```python
from build123d import *

# Parameters (mm, degrees)
ESQUISSE1_W                  = 52
ESQUISSE1_H                  = 3
CHANFREIN1_SIZE              = 0.5
ENL_V_MAT_EXTRU_1_DEPTH      = 27.343879745
ENL_V_MAT_EXTRU_1_DEPTH_BACK = 27.343879745
ESQUISSE2_W                  = 4
ESQUISSE2_H                  = 2
ESQUISSE3_W                  = 0.74
ESQUISSE3_H                  = 1
BOSS_EXTRU_1_START           = 15
ESQUISSE4_R                  = 3
BOSS_EXTRU_1_DEPTH           = 15
ENL_V_MAT_EXTRU_2_DEPTH      = 42.218927691
ENL_V_MAT_EXTRU_2_DEPTH_BACK = 42.218927691
ESQUISSE5_W                  = 12
ESQUISSE5_H                  = 1
ENL_V_MAT_EXTRU_3_DEPTH      = 42.218927691
ENL_V_MAT_EXTRU_3_DEPTH_BACK = 42.218927691
ESQUISSE6_W                  = 50.211323454
ESQUISSE6_H                  = 20.21753951


with BuildPart() as part:
    # Esquisse1 → Révolution1 (revolve)
    with BuildSketch(Plane.XY, mode=Mode.PRIVATE) as r_volution1_sk:
        with Locations((0, 1.5)):
            Rectangle(ESQUISSE1_W, ESQUISSE1_H)
    revolve(r_volution1_sk.sketch.rotate(Axis((0, 0, 0), (1, 0, 0)), 90), axis=Axis((0, 0, 0), (1, 0, 0)))

    # Chanfrein1
    chanfrein1_edges = [part.edges().sort_by_distance(p)[0] for p in [
        (26, 0, -3),
    ]]
    chamfer(chanfrein1_edges, length=CHANFREIN1_SIZE)

    # Esquisse2 → Enlèv. mat.-Extru.1 (cut, two sides: drawn at the far end of the back side and taken through both)
    with BuildSketch(Plane.XY.offset(-ENL_V_MAT_EXTRU_1_DEPTH_BACK)):
        with Locations((9.5, 3)):
            Rectangle(ESQUISSE2_W, ESQUISSE2_H)
    extrude(amount=ENL_V_MAT_EXTRU_1_DEPTH + ENL_V_MAT_EXTRU_1_DEPTH_BACK, mode=Mode.SUBTRACT)

    # Esquisse3 → Enlèvement de matière-Révolution1 (revolve, cut)
    with BuildSketch(Plane.XY):
        with Locations((-21.03, 2.5)):
            Rectangle(ESQUISSE3_W, ESQUISSE3_H)
        with Locations((21.03, 2.5)):
            Rectangle(ESQUISSE3_W, ESQUISSE3_H)
    revolve(axis=Axis((0, 0, 0), (-1, 0, 0)), mode=Mode.SUBTRACT)

    # Esquisse4 → Boss.-Extru.1 (add)
    with BuildSketch(Plane.ZY.offset(26).offset(BOSS_EXTRU_1_START)):
        with Locations(Location((0, 0, 0), (0, 0, 90))):
            Circle(ESQUISSE4_R)
    extrude(amount=-BOSS_EXTRU_1_DEPTH)

    # Esquisse5 → Enlèv. mat.-Extru.2 (cut, two sides: drawn at the far end of the back side and taken through both)
    with BuildSketch(Plane.XY.offset(-ENL_V_MAT_EXTRU_2_DEPTH_BACK)):
        with Locations((-35, 2.5)):
            Rectangle(ESQUISSE5_W, ESQUISSE5_H)
    extrude(amount=ENL_V_MAT_EXTRU_2_DEPTH + ENL_V_MAT_EXTRU_2_DEPTH_BACK, mode=Mode.SUBTRACT)

    # Esquisse6 → Enlèv. mat.-Extru.3 (cut, two sides: drawn at the far end of the back side and taken through both)
    with BuildSketch(Plane.XY.offset(-ENL_V_MAT_EXTRU_3_DEPTH_BACK)):
        with Locations((-25.105661727, 1.097333559)):
            Rectangle(ESQUISSE6_W, ESQUISSE6_H)
    extrude(amount=ENL_V_MAT_EXTRU_3_DEPTH + ENL_V_MAT_EXTRU_3_DEPTH_BACK, mode=Mode.SUBTRACT)


solid = part.part
```
The listing builds one solid part. Answer for the finished solid, in the listing's coordinates (mm). A direction names the side the tool comes from. Coordinates: 2 decimals unless noted, no trailing zeros. Write each loop counter-clockwise with the first axis right and the second up, starting at its lowest first coordinate (ties: lowest second). Pieces come first, ordered by that corner, then holes.
Q1. Section B-B, the plane x = 17 is taken. Write down the section's boundary in (y, z).
Returned:
outline: circle Ø6 at (0, 0)
Q2. Given P1, Ø1.5, axis at x = 12, y = 1, coming from the -Z side; P2, Ø3, axis at y = 1, z = 0.5, coming from the -X side; P3, Ø2, axis at x = 10, z = 1, coming from the +Y side; P4, Ø2, axis at x = 22.5, y = -2, coming from the -Z side, each flat-ended and moving along its own axis, determine where each tip first touches the part or whether it passes through.
Returned:
P1: stops at z = -2.99
P2: stops at x = 0
P3: stops at y = 2
P4: stops at z = -2.83
Q3. Section C-C, the plane x = 10 is taken. Write down the section's boundary in (y, z), then the cut area to 3 significant figures.
Returned:
outline: (2, -2.24) - (2, 2.24) arc R3 ccw (long way) to start
area: 25.2 mm2
Q4. Section A-A, the plane z = 0 is taken. Write down the section's boundary in (x, y).
Returned:
outline: (0, -3) - (20.66, -3) - (20.66, -2) - (21.4, -2) - (21.4, -3) - (25.5, -3) - (26, -2.5) - (26, 2.5) - (25.5, 3) - (21.4, 3) - (21.4, 2) - (20.66, 2) - (20.66, 3) - (11.5, 3) - (11.5, 2) - (7.5, 2) - (7.5, 3) - (0, 3) - close
Q5. Which of the six approach directions +Z, -Z, +X, -X, +Y, -Y give full straight-line access (tool end or side, diameter ignored) to faces 5 (the flat face through (11.5, 2.4, 0)), 6 (the cylindrical face through (23.48, 1.15, 2.77)), 7 (the cylindrical face through (21, 0, 2))?
Returned:
face 5: +Z, -Z, +Y
face 6: +X, -X
face 7: none
Q6. The mould has two halves that part along X. Classify faces 1 (the flat face through (20.66, -1, 2)), 2 (the flat face through (0, 0, 0)), 3 (the flat face through (26, 0, 0)), 4 (the cylindrical face through (10, -3, 0)): released by +X, released by -X, zero draft, split by the parting line, or undercut.
Returned:
face 1: undercut
face 2: released by -X
face 3: released by +X
face 4: zero draft
Q7. Find the intervals of material crossed by line 1 along X through (y, z) = (-0.2, -2.3); line 2 along X through (y, z) = (-0.1, -2.6); line 3 along Z through (x, y) = (5.25, 1.5), in increasing order.
Returned:
line 1: x = 0 to 20.66, 21.4 to 26
line 2: x = 0 to 20.66, 21.4 to 25.9
line 3: z = -2.6 to 2.6
